For this review, use the dimensioned drawing (mm, ordinates from the lowest corner) and the shaded views. A direction names the side the tool comes from. Give positions to 0.01 mm unless a question says otherwise; leave off trailing zeros. Order: outer loops, then holes, each group sorted by start corner. A loop starts at its lowest first (then second) coordinate and runs counter-clockwise, first axis right, second up. Notation, with made-up numbers: M -7.75,-14 L 16.25,-14 A15 ccw 16.25,5 Z; hole C 84,48.25 d10. An arc over 180 degrees is marked long. Answer as CSV lines item,"result". Start each with the question number.
1. Mouldability with a two-part tool opening along X and no side actions: class the marked faces 3, 4 and 5 as pulls with the +X half, pulls with the -X half, needs draft (parallel to the pull), parting line crosses it, or undercut.
2. We need section A-A, the plane y = 29. Give the boundary of the cut face in (x, z), and give its area (3 significant figures).
3. We need section C-C, the plane y = 6. Give the boundary of the cut face in (x, z), and give its area (3 significant figures).
4. For line 1 along X through (y, z) = (26.5, 21.5); line 2 along Z through (x, y) = (4, 13); line 3 along X through (y, z) = (38, 9.75), list the stretches that pass through material, from the lowest coordinate up.
5. Clearance check with flat-ended pins moving along their axes: P1, Ø12, axis at x = 12.5, z = 17.5, coming from the -Y side; P2, Ø12, axis at x = 28.5, z = 18, coming from the -Y side; P3, Ø1, axis at y = 42.5, z = 9, coming from the +X side. State where each tip first meets the part, or that it passes through.
6. We need section D-D, the plane z = 14.5. Give the boundary of the cut face in (x, y) (3 decimals).
7. We need section B-B, the plane x = 39. Give the boundary of the cut face in (y, z), and give its area (3 significant figures).
8. Machinability: for the marked faces 1 and 2, which of the approach directions +Z, -Z, +X, -X, +Y, -Y give a long, thin tool a straight path to every point of the face, cutting with its end or side? Answer none if there is none.
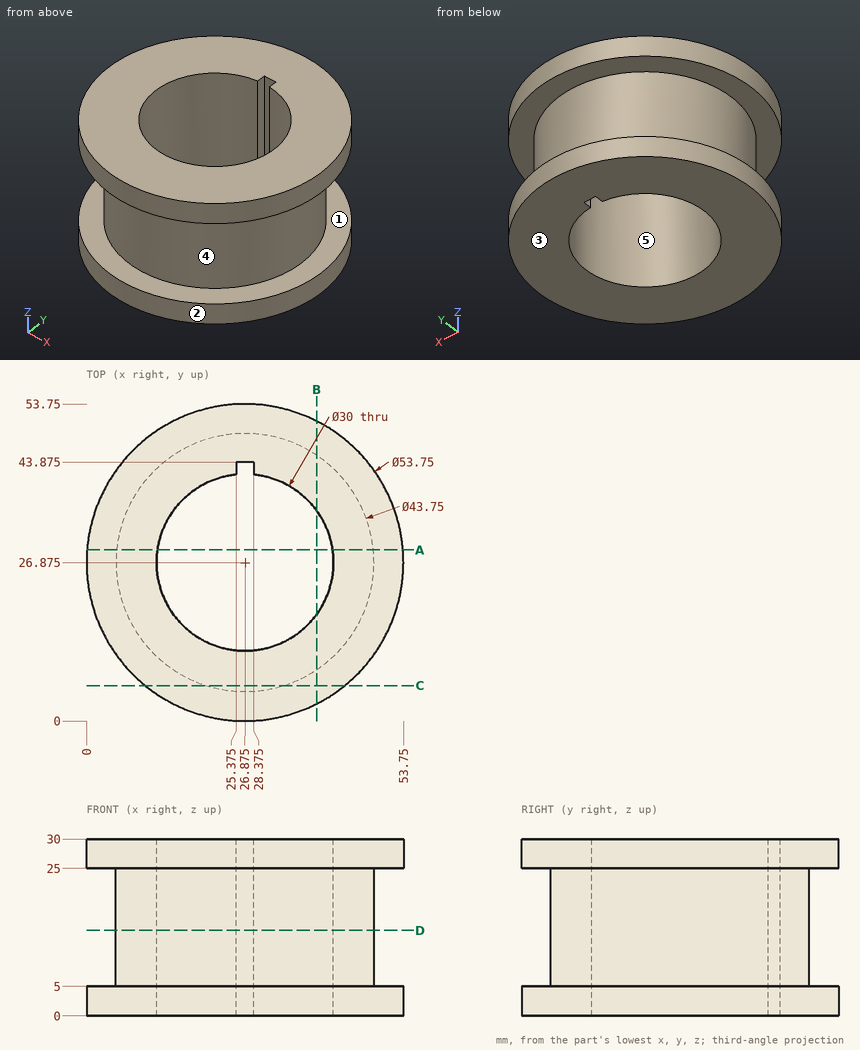
Result set:
1,face 3,"needs draft"
1,face 4,"parting line crosses it"
1,face 5,"undercut"
2,outline,"M 0.08,0 L 12.03,0 L 12.03,30 L 0.08,30 L 0.08,25 L 5.1,25 L 5.1,5 L 0.08,5 Z; M 41.72,0 L 53.67,0 L 53.67,5 L 48.65,5 L 48.65,25 L 53.67,25 L 53.67,30 L 41.72,30 Z"
2,area,"516 mm2"
3,outline,"M 9.95,0 L 43.8,0 L 43.8,5 L 33.41,5 L 33.41,25 L 43.8,25 L 43.8,30 L 9.95,30 L 9.95,25 L 20.34,25 L 20.34,5 L 9.95,5 Z"
3,area,"600 mm2"
4,line 1,"5 to 11.88, 41.87 to 48.75"
4,line 2,"0 to 5, 25 to 30"
4,line 3,"8.04 to 16.81, 36.94 to 45.71"
5,P1,"y = 6.67"
5,P2,"y = 5"
5,P3,"x = 42.68"
6,outline,"C 26.875,26.875 d43.75; hole M 25.375,41.8 A15 ccw long 28.375,41.8 L 28.375,43.875 L 25.375,43.875 Z"
7,outline,"M 2.89,0 L 18.04,0 L 18.04,30 L 2.89,30 L 2.89,25 L 8.67,25 L 8.67,5 L 2.89,5 Z; M 35.71,0 L 50.86,0 L 50.86,5 L 45.08,5 L 45.08,25 L 50.86,25 L 50.86,30 L 35.71,30 Z"
7,area,"678 mm2"
8,face 1,"none"
8,face 2,"+Z, -Z"
